Part print with two shaded views. Sizes in mm from the minimum x, y, z corner. Round coordinates to 2 decimals unless told otherwise and drop trailing zeros. Write each loop counter-clockwise with the first axis right and the second up, starting at its lowest first coordinate (ties: lowest second). Pieces come first, ordered by that corner, then holes. Notation, with made-up numbers: M -17,-2 L 9,-2 A20 cw 9,36 Z; hole C -30,-12.75 d4. An arc over 180 degrees is marked long. Use one line per item in the form item = value. Start each with the question number.
Item 1: Probe L1, parallel to Y at x = 78.15, z = 4.5; L2, parallel to X at y = 2.5, z = 2; L3, parallel to Z at x = 41, y = 8.5. List the from-to ranges inside material, lowest first.
Item 2: Flat gauge pins, fed straight in: pin 1 Ø1.3 at (x, z) = (2, 5) entering from +Y; pin 2 Ø1 at (x, y) = (1.5, 33.5) entering from +Z; pin 3 Ø3 at (x, y) = (53, 16) entering from -Z; pin 4 Ø1 at (x, y) = (51.5, 6.5) entering from +Z. Where does each tip first touch, or does it go through?
Item 3: Cut at B-B, the plane z = 4.5. Give the cut face in (x, y).
Item 4: Cut at A-A, the plane y = 19. Give the cut face in (x, z), then the cut area to 3 significant figures.
Item 5: Cut at C-C, the plane y = 4. Give the cut face in (x, z).
Item 6: Cut at D-D, the plane x = 41.5. Give the cut face in (y, z), then the cut area to 3 significant figures.
Item 7: Mould opens along X. For the marked faces 1 and 2 say: +X half, -X half, draft (parallel to the pull), parting line (faces both ways), or undercut.
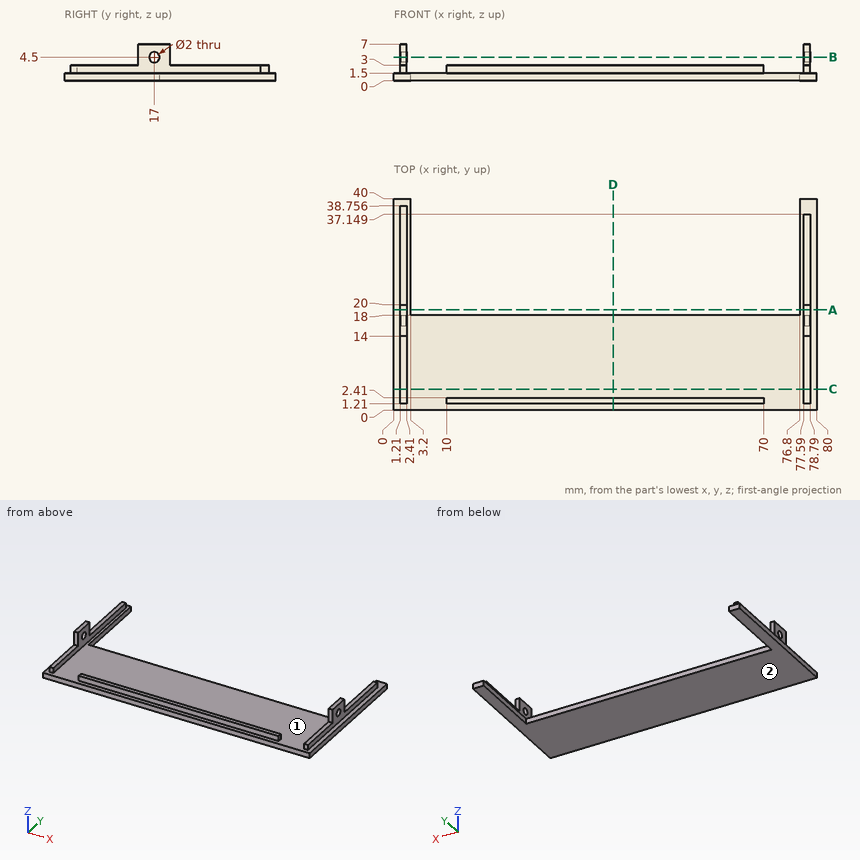
Model answer:
q1.L1 = 14 to 16, 18 to 20
q1.L2 = 1.21 to 2.41, 77.59 to 78.79
q1.L3 = 0 to 1.5
q2.pin_1 = 20
q2.pin_2 = 3
q2.pin_3 = 0
q2.pin_4 = 1.5
q3.outline = M 1.21,14 L 2.41,14 L 2.41,16 L 1.21,16 Z; M 1.21,18 L 2.41,18 L 2.41,20 L 1.21,20 Z; M 77.59,14 L 78.79,14 L 78.79,16 L 77.59,16 Z; M 77.59,18 L 78.79,18 L 78.79,20 L 77.59,20 Z
q4.outline = M 0,0 L 3.2,0 L 3.2,1.5 L 2.41,1.5 L 2.41,7 L 1.21,7 L 1.21,1.5 L 0,1.5 Z; M 76.8,0 L 80,0 L 80,1.5 L 78.79,1.5 L 78.79,7 L 77.59,7 L 77.59,1.5 L 76.8,1.5 Z
q4.area = 22.8 mm²
q5.outline = M 0,0 L 80,0 L 80,1.5 L 78.79,1.5 L 78.79,3 L 77.59,3 L 77.59,1.5 L 2.41,1.5 L 2.41,3 L 1.21,3 L 1.21,1.5 L 0,1.5 Z
q6.outline = M 0,0 L 18,0 L 18,1.5 L 2.41,1.5 L 2.41,3 L 1.21,3 L 1.21,1.5 L 0,1.5 Z
q6.area = 28.8 mm²
q7.face_1 = undercut
q7.face_2 = draft
